Input: part model. Units: mm. Frame: model coordinates. Give positions to 0.01 mm unless a question says otherwise; leave off trailing zeros. Order: outer loops, then holes, each group sorted by start corner. A loop starts at its lowest first (then second) coordinate and runs counter-clockwise, first axis right, second up.
```python
from build123d import *

# Parameters (mm, degrees)
BOSS_EXTRUDE1_DEPTH = 8
CUT_EXTRUDE1_DEPTH  = 90
SKETCH3_R           = 5
CUT_EXTRUDE2_DEPTH  = 5.4
SKETCH5_R           = 10.3
CUT_EXTRUDE3_DEPTH  = 20
SKETCH7_R           = 20.6
SKETCH7_R_2         = 15.6
CUT_EXTRUDE5_DEPTH  = 2.5
CUT_EXTRUDE6_REACH  = 127.974
SKETCH9_R           = 6.575
SKETCH9_R_2         = 2.1
SKETCH9_R_3         = 1.025
SKETCH10_R          = 2.1
CUT_EXTRUDE10_DEPTH = 10
CUT_EXTRUDE11_DEPTH = 2.5
BOSS_EXTRUDE2_START = -1
SKETCH12_R          = 1.025
BOSS_EXTRUDE2_DEPTH = 1
FILLET1_R           = 0.5


with BuildPart() as part:
    # Sketch1 → Boss-Extrude1 (new body)
    with BuildSketch(Plane.XY):
        with BuildLine():
            Line((-83.790627288, -89.5), (83.790627288, -89.5))
            ThreePointArc((83.790627288, -89.5), (86.972607803, -88.181980515), (88.290627288, -85))
            Line((88.290627288, -85), (88.290627288, 85))
            ThreePointArc((88.290627288, 85), (86.972607803, 88.181980515), (83.790627288, 89.5))
            Line((83.790627288, 89.5), (-83.790627288, 89.5))
            ThreePointArc((-83.790627288, 89.5), (-86.972607803, 88.181980515), (-88.290627288, 85))
            Line((-88.290627288, 85), (-88.290627288, -85))
            ThreePointArc((-88.290627288, -85), (-86.972607803, -88.181980515), (-83.790627288, -89.5))
        make_face()
    extrude(amount=BOSS_EXTRUDE1_DEPTH)

    # Sketch2 → Cut-Extrude1 (cut)
    with BuildSketch(Plane.XY.offset(8)):
        with BuildLine():
            ThreePointArc((43.745313644, 83.5), (41.145313644, 86.1), (38.545313644, 83.5))
            ThreePointArc((38.545313644, 83.5), (41.145313644, 80.9), (43.745313644, 83.5))
        make_face()
        with BuildLine():
            Line((0, 84), (2.551470164, 84))
            ThreePointArc((2.551470164, 84), (0, 86.1), (-2.551470164, 84))
            Line((-2.551470164, 84), (0, 84))
        make_face()
        with BuildLine():
            Line((0, 84), (-2.551470164, 84))
            ThreePointArc((-2.551470164, 84), (0, 80.9), (2.551470164, 84))
            Line((2.551470164, 84), (0, 84))
        make_face()
        with BuildLine():
            ThreePointArc((-43.745313644, 83.5), (-41.145313644, 80.9), (-38.545313644, 83.5))
            ThreePointArc((-38.545313644, 83.5), (-41.145313644, 86.1), (-43.745313644, 83.5))
        make_face()
        with BuildLine():
            ThreePointArc((-84.890627288, 83.5), (-82.290627288, 80.9), (-79.690627288, 83.5))
            ThreePointArc((-79.690627288, 83.5), (-82.290627288, 86.1), (-84.890627288, 83.5))
        make_face()
        with BuildLine():
            ThreePointArc((-84.890627288, 41.75), (-82.290627288, 39.15), (-79.690627288, 41.75))
            ThreePointArc((-79.690627288, 41.75), (-82.290627288, 44.35), (-84.890627288, 41.75))
        make_face()
        with BuildLine():
            ThreePointArc((-84.890627288, 0), (-82.290627288, -2.6), (-79.690627288, 0))
            ThreePointArc((-79.690627288, 0), (-82.290627288, 2.6), (-84.890627288, 0))
        make_face()
        with BuildLine():
            ThreePointArc((-79.690627288, -83.5), (-82.290627288, -80.9), (-84.890627288, -83.5))
            ThreePointArc((-84.890627288, -83.5), (-82.290627288, -86.1), (-79.690627288, -83.5))
        make_face()
        with BuildLine():
            ThreePointArc((-84.890627288, -41.75), (-82.290627288, -44.35), (-79.690627288, -41.75))
            ThreePointArc((-79.690627288, -41.75), (-82.290627288, -39.15), (-84.890627288, -41.75))
        make_face()
        with BuildLine():
            ThreePointArc((-43.745313644, -83.5), (-41.145313644, -86.1), (-38.545313644, -83.5))
            ThreePointArc((-38.545313644, -83.5), (-41.145313644, -80.9), (-43.745313644, -83.5))
        make_face()
        with BuildLine():
            ThreePointArc((-2.6, -83.5), (0, -86.1), (2.6, -83.5))
            ThreePointArc((2.6, -83.5), (0, -80.9), (-2.6, -83.5))
        make_face()
        with BuildLine():
            ThreePointArc((38.545313644, -83.5), (41.145313644, -86.1), (43.745313644, -83.5))
            ThreePointArc((43.745313644, -83.5), (41.145313644, -80.9), (38.545313644, -83.5))
        make_face()
        with BuildLine():
            ThreePointArc((79.690627288, -83.5), (82.290627288, -86.1), (84.890627288, -83.5))
            ThreePointArc((84.890627288, -83.5), (82.290627288, -80.9), (79.690627288, -83.5))
        make_face()
        with BuildLine():
            ThreePointArc((79.690627288, -41.75), (82.290627288, -44.35), (84.890627288, -41.75))
            ThreePointArc((84.890627288, -41.75), (82.290627288, -39.15), (79.690627288, -41.75))
        make_face()
        with BuildLine():
            ThreePointArc((79.690627288, 0), (82.290627288, -2.6), (84.890627288, 0))
            ThreePointArc((84.890627288, 0), (82.290627288, 2.6), (79.690627288, 0))
        make_face()
        with BuildLine():
            ThreePointArc((79.690627288, 41.75), (82.290627288, 39.15), (84.890627288, 41.75))
            ThreePointArc((84.890627288, 41.75), (82.290627288, 44.35), (79.690627288, 41.75))
        make_face()
        with BuildLine():
            ThreePointArc((79.690627288, 83.5), (82.290627288, 80.9), (84.890627288, 83.5))
            ThreePointArc((84.890627288, 83.5), (82.290627288, 86.1), (79.690627288, 83.5))
        make_face()
    extrude(amount=-CUT_EXTRUDE1_DEPTH, mode=Mode.SUBTRACT)

    # Sketch3 → Cut-Extrude2 (cut)
    with BuildSketch(Plane.XY.offset(8)):
        with Locations((41.145313644, 83.5)):
            Circle(SKETCH3_R)
        with Locations((82.290627288, 83.5)):
            Circle(SKETCH3_R)
        with Locations((82.290627288, 41.75)):
            Circle(SKETCH3_R)
        with Locations((82.290627288, 0)):
            Circle(SKETCH3_R)
        with Locations((82.290627288, -41.75)):
            Circle(SKETCH3_R)
        with Locations((82.290627288, -83.5)):
            Circle(SKETCH3_R)
        with Locations((41.145313644, -83.5)):
            Circle(SKETCH3_R)
        with Locations((0, -83.5)):
            Circle(SKETCH3_R)
        with Locations((-82.290627288, 0)):
            Circle(SKETCH3_R)
        with Locations((-82.290627288, -83.5)):
            Circle(SKETCH3_R)
        with Locations((-82.290627288, -41.75)):
            Circle(SKETCH3_R)
        with Locations((-41.145313644, -83.5)):
            Circle(SKETCH3_R)
        with Locations((-82.290627288, 41.75)):
            Circle(SKETCH3_R)
        with Locations((-82.290627288, 83.5)):
            Circle(SKETCH3_R)
        with Locations((-41.145313644, 83.5)):
            Circle(SKETCH3_R)
        with Locations((0, 83.5)):
            Circle(SKETCH3_R)
    extrude(amount=-CUT_EXTRUDE2_DEPTH, mode=Mode.SUBTRACT)

    # Sketch5 → Cut-Extrude3 (cut)
    with BuildSketch(Plane.XY.offset(8)):
        with Locations((33.49662103, -33.754772237)):
            Circle(SKETCH5_R)
    extrude(amount=-CUT_EXTRUDE3_DEPTH, mode=Mode.SUBTRACT)

    # Sketch7 → Cut-Extrude5 (cut)
    with BuildSketch(Plane.XY.offset(8)):
        with Locations((-32.990627288, -34.2)):
            Circle(SKETCH7_R)
        with Locations((-32.990627288, -34.2)):
            Circle(SKETCH7_R_2, mode=Mode.SUBTRACT)
    extrude(amount=-CUT_EXTRUDE5_DEPTH, mode=Mode.SUBTRACT)

    # Sketch9 → Cut-Extrude6 (cut, up to next)
    with BuildSketch(Plane.XY.offset(8), mode=Mode.PRIVATE) as cut_extrude6_sk1:
        with Locations((-32.990627288, -34.2)):
            Circle(SKETCH9_R)
    cut_extrude6_tool1 = extrude(cut_extrude6_sk1.sketch, amount=-CUT_EXTRUDE6_REACH, mode=Mode.PRIVATE) & part.part
    # Sketch9 → Cut-Extrude6 (cut, up to next)
    with BuildSketch(Plane.XY.offset(8), mode=Mode.PRIVATE) as cut_extrude6_sk2:
        with Locations((-32.990627288, -5.7)):
            Circle(SKETCH9_R_2)
    cut_extrude6_tool2 = extrude(cut_extrude6_sk2.sketch, amount=-CUT_EXTRUDE6_REACH, mode=Mode.PRIVATE) & part.part
    # Sketch9 → Cut-Extrude6 (cut, up to next)
    with BuildSketch(Plane.XY.offset(8), mode=Mode.PRIVATE) as cut_extrude6_sk3:
        with Locations((-32.990627288, -23.0748)):
            Circle(SKETCH9_R_3)
    cut_extrude6_tool3 = extrude(cut_extrude6_sk3.sketch, amount=-CUT_EXTRUDE6_REACH, mode=Mode.PRIVATE) & part.part
    # Sketch9 → Cut-Extrude6 (cut, up to next)
    with BuildSketch(Plane.XY.offset(8), mode=Mode.PRIVATE) as cut_extrude6_sk4:
        with Locations((-32.990627288, -45.3252)):
            Circle(SKETCH9_R_3)
    cut_extrude6_tool4 = extrude(cut_extrude6_sk4.sketch, amount=-CUT_EXTRUDE6_REACH, mode=Mode.PRIVATE) & part.part
    # Sketch9 → Cut-Extrude6 (cut, up to next)
    with BuildSketch(Plane.XY.offset(8), mode=Mode.PRIVATE) as cut_extrude6_sk5:
        with Locations((-4.490627288, -34.2)):
            Circle(SKETCH9_R_2)
    cut_extrude6_tool5 = extrude(cut_extrude6_sk5.sketch, amount=-CUT_EXTRUDE6_REACH, mode=Mode.PRIVATE) & part.part
    # Sketch9 → Cut-Extrude6 (cut, up to next)
    with BuildSketch(Plane.XY.offset(8), mode=Mode.PRIVATE) as cut_extrude6_sk6:
        with Locations((-32.990627288, -62.7)):
            Circle(SKETCH9_R_2)
    cut_extrude6_tool6 = extrude(cut_extrude6_sk6.sketch, amount=-CUT_EXTRUDE6_REACH, mode=Mode.PRIVATE) & part.part
    # Sketch9 → Cut-Extrude6 (cut, up to next)
    with BuildSketch(Plane.XY.offset(8), mode=Mode.PRIVATE) as cut_extrude6_sk7:
        with Locations((-61.490627288, -34.2)):
            Circle(SKETCH9_R_2)
    cut_extrude6_tool7 = extrude(cut_extrude6_sk7.sketch, amount=-CUT_EXTRUDE6_REACH, mode=Mode.PRIVATE) & part.part
    add(cut_extrude6_tool1.solids().sort_by_distance((-32.990627, -34.2, 8))[0], mode=Mode.SUBTRACT)
    add(cut_extrude6_tool2.solids().sort_by_distance((-32.990627, -5.7, 8))[0], mode=Mode.SUBTRACT)
    add(cut_extrude6_tool3.solids().sort_by_distance((-32.990627, -23.0748, 8))[0], mode=Mode.SUBTRACT)
    add(cut_extrude6_tool4.solids().sort_by_distance((-32.990627, -45.3252, 8))[0], mode=Mode.SUBTRACT)
    add(cut_extrude6_tool5.solids().sort_by_distance((-4.490627, -34.2, 8))[0], mode=Mode.SUBTRACT)
    add(cut_extrude6_tool6.solids().sort_by_distance((-32.990627, -62.7, 8))[0], mode=Mode.SUBTRACT)
    add(cut_extrude6_tool7.solids().sort_by_distance((-61.490627, -34.2, 8))[0], mode=Mode.SUBTRACT)

    # Sketch10 → Cut-Extrude10 (cut)
    with BuildSketch(Plane.XY.offset(8)):
        with Locations((54.971257232, -21.754772237)):
            Circle(SKETCH10_R)
        with Locations((41.99662103, -10.669928724)):
            Circle(SKETCH10_R)
        with Locations((24.99662103, -10.669928724)):
            Circle(SKETCH10_R)
        with Locations((12.021984828, -21.754772237)):
            Circle(SKETCH10_R)
        with Locations((12.021984828, -45.754772237)):
            Circle(SKETCH10_R)
        with Locations((24.99662103, -56.839615749)):
            Circle(SKETCH10_R)
        with Locations((41.99662103, -56.839615749)):
            Circle(SKETCH10_R)
        with Locations((54.971257232, -45.754772237)):
            Circle(SKETCH10_R)
    extrude(amount=-CUT_EXTRUDE10_DEPTH, mode=Mode.SUBTRACT)

    # Sketch11 → Cut-Extrude11 (cut)
    with BuildSketch(Plane.XY.offset(8)):
        with BuildLine():
            ThreePointArc((33.49662103, -20.654772237), (20.39662103, -33.754772237), (33.49662103, -46.854772237))
            ThreePointArc((33.49662103, -46.854772237), (46.59662103, -33.754772237), (33.49662103, -20.654772237))
        make_face()
    extrude(amount=-CUT_EXTRUDE11_DEPTH, mode=Mode.SUBTRACT)

    # Sketch12 → Boss-Extrude2 (add)
    with BuildSketch(Plane(origin=(0, 0, 0), x_dir=(-1, 0, 0), z_dir=(0, 0, -1)).offset(BOSS_EXTRUDE2_START)):
        with Locations(Location((32.990627288, -23.0748, 0), (0, 0, 180))):
            Circle(SKETCH12_R)
        with Locations(Location((32.990627288, -45.3252, 0), (0, 0, 180))):
            Circle(SKETCH12_R)
    extrude(amount=BOSS_EXTRUDE2_DEPTH)

    # Fillet1
    fillet1_edges = [part.edges().sort_by_distance(p)[0] for p in [
        (-34.015627288, -23.0748, 1),
        (-34.015627288, -45.3252, 1),
    ]]
    fillet(fillet1_edges, radius=FILLET1_R)


solid = part.part
```
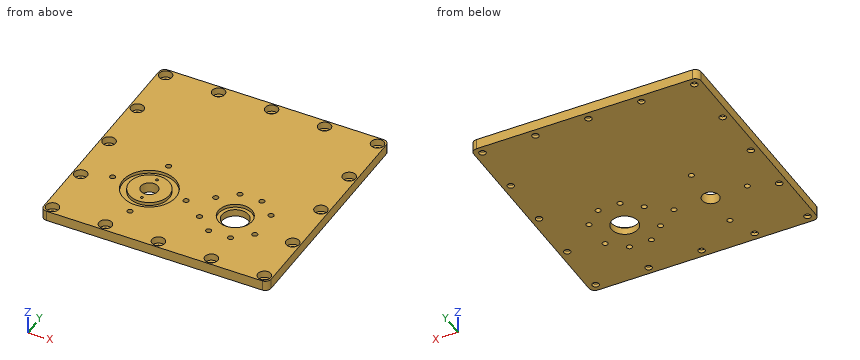
1) Cut plane D-D (z = 4). Count the separate pieces of the cut face and the enclosed holes in it, then the cut area to 3 significant figures.
2) Cut plane A-A (x = 0). Return the cut outline in (y, z).
3) Cut plane B-B (y = 41.75). Return the cut outline in (x, z).
4) First-contact query: P1, Ø3, axis at x = -82.29, y = -83.5, coming from the -Z side; P2, Ø6, axis at x = 67.5, y = 26.5, coming from the -Z side; P3, Ø3, axis at x = 81.5, y = -86, coming from the +Z side. Flat tips, straight axial feed; report the tip coordinate or a pass-through.
5) Line query: probe 1 along Y at (x, z) = (78, 7); probe 2 along Y at (x, z) = (0, 6.7); probe 3 along X at (y, z) = (-12.5, 6.5). Output: solid intervals per line, ascending.
6) Cut plane C-C (y = -62.7). Return the cut outline in (x, z), then the cut area to 3 significant figures.
Geometry says:
1. separate pieces: 1
1. enclosed holes: 32
1. area: 29,700 mm2
2. outline: (-89.5, 0) - (-86.1, 0) - (-86.1, 2.6) - (-88.5, 2.6) - (-88.5, 8) - (-89.5, 8) - close; (-80.9, 0) - (80.9, 0) - (80.9, 2.6) - (78.5, 2.6) - (78.5, 8) - (-78.5, 8) - (-78.5, 2.6) - (-80.9, 2.6) - close; (86.1, 0) - (89.5, 0) - (89.5, 8) - (88.5, 8) - (88.5, 2.6) - (86.1, 2.6) - close
3. outline: (-88.29, 0) - (-84.89, 0) - (-84.89, 2.6) - (-87.29, 2.6) - (-87.29, 8) - (-88.29, 8) - close; (-79.69, 0) - (79.69, 0) - (79.69, 2.6) - (77.29, 2.6) - (77.29, 8) - (-77.29, 8) - (-77.29, 2.6) - (-79.69, 2.6) - close; (84.89, 0) - (88.29, 0) - (88.29, 8) - (87.29, 8) - (87.29, 2.6) - (84.89, 2.6) - close
4. P1: passes through
4. P2: stops at z = 0
4. P3: stops at z = 2.6
5. probe 1: y = -89.5 to -86.07, -80.93 to -44.32, -39.18 to -2.57, 2.57 to 39.18, 44.32 to 80.93, 86.07 to 89.5
5. probe 2: y = -89.5 to -88.5, -78.5 to 78.5, 88.5 to 89.5
5. probe 3: x = -88.29 to 23.97, 26.03 to 40.97, 43.03 to 88.29
6. outline: (-88.29, 0) - (-35.09, 0) - (-35.09, 8) - (-88.29, 8) - close; (-30.89, 0) - (88.29, 0) - (88.29, 8) - (-30.89, 8) - close
6. area: 1,380 mm2
